The drawing under review shows one solid part. Ordinate dimensions are in mm from its lowest x, y, z. A direction names the side the tool comes from. Give positions to 0.01 mm unless a question says otherwise; leave off trailing zeros. Write each loop counter-clockwise with the first axis right and the second up, starting at its lowest first coordinate (ties: lowest second). Pieces come first, ordered by that corner, then holes. Notation, with made-up numbers: (88.25, 6) -> (139.25, 6) arc R21 ccw to (139.25, 12) -> close; hole circle Ø9 at (68.5, 61.25). An arc over 180 degrees is marked (long way). Write item = value, one per line.
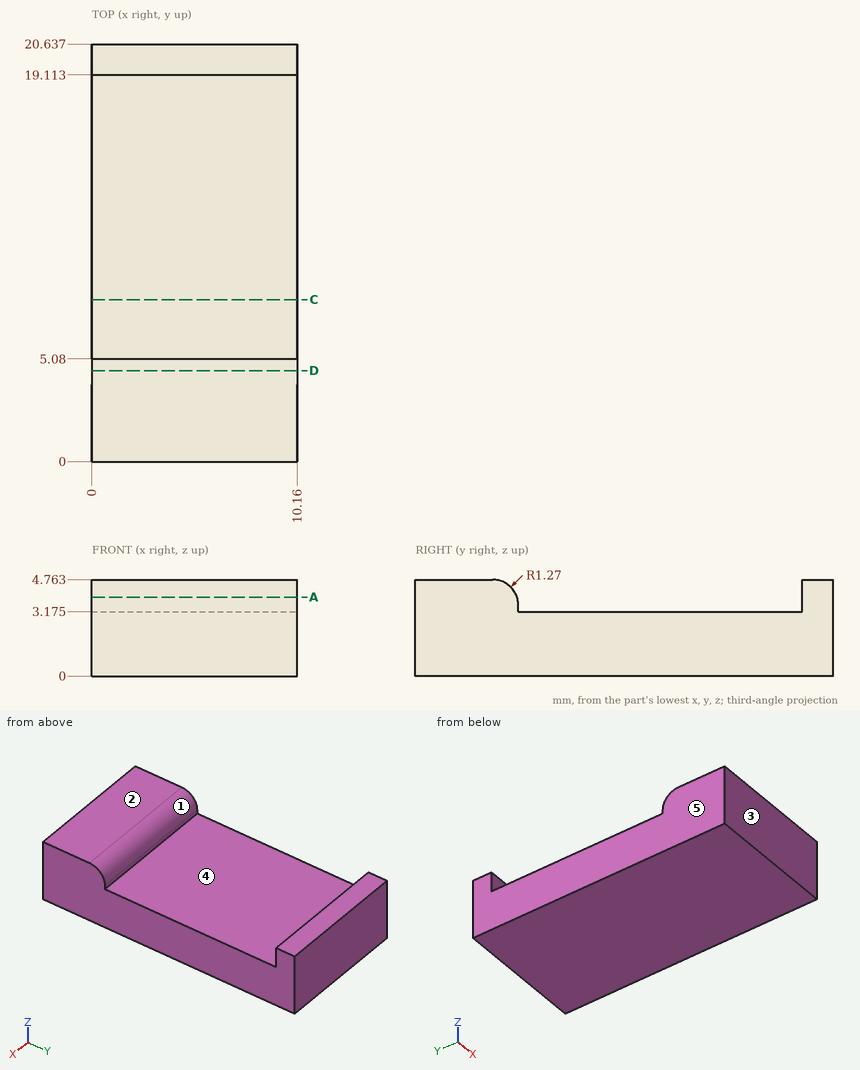
(1) The part is to be moulded in two halves that separate along Y. For the marked faces 3, 4 and 5, say which applies: released by +Y, released by -Y, zero draft, split by the parting line, or undercut.
Answers below:
face_3 = released by -Y
face_4 = undercut
face_5 = zero draft
(2) For pin 1 (4 mm diameter, centred on x = 2.5, y = 4, fed in from +Z); pin 2 (4 mm diameter, centred on x = 5.5, y = 14, fed in from +Z) (1 decimal), all flat-tipped, find the tip position at first contact; note any pin that passes through.
Answers below:
pin_1 = 4.76
pin_2 = 3.2
(3) Take a section at D-D (y = 4.5). Write out the cut boundary in (x, z), plus the area to 3 significant figures.
Answers below:
outline = (0, 0) -> (10.16, 0) -> (10.16, 4.56) -> (0, 4.56) -> close
area = 46.3 mm^2
(4) Tool access review of the marked faces 1 and 2: name each direction out of +Z, -Z, +X, -X, +Y, -Y from which nothing blocks a thin tool from reaching the whole face with its end or side.
Answers below:
face_1 = +Z, +X, -X
face_2 = +Z, +X, -X, +Y, -Y
(5) Take a section at A-A (z = 3.9). Write out the cut boundary in (x, y).
Answers below:
outline = (0, 0) -> (10.16, 0) -> (10.16, 5.01) -> (0, 5.01) -> close; (0, 19.11) -> (10.16, 19.11) -> (10.16, 20.64) -> (0, 20.64) -> close
(6) To check wall thickness, follow probe 1 along Y at (x, z) = (8.5, 3.6) (1 decimal); probe 2 along Z at (x, y) = (5.5, 9.25) (1 decimal). State the ranges of each line that lie inside material, in increasing order.
Answers below:
probe_1 = 0 to 5.1, 19.1 to 20.6
probe_2 = 0 to 3.2
(7) Take a section at C-C (y = 8). Write out the cut boundary in (x, z) (1 decimal).
Answers below:
outline = (0, 0) -> (10.2, 0) -> (10.2, 3.2) -> (0, 3.2) -> close
